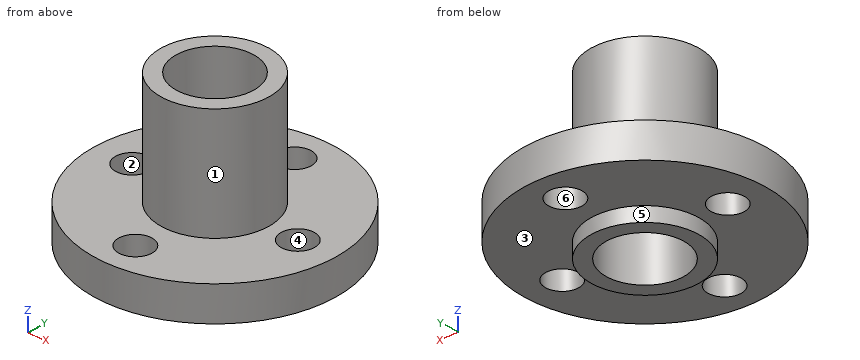
Autodesk Fusion 360 part; units mm, degrees
sketch "Sketch1" plane through (0, 0, 0) normal (0, 0, 1) x (1, 0, 0)
  circle A0 centre (0, 0) radius 10.9
  dimension "d1" = 21.8
extrude "Extrude1" add sketch "Sketch1" along normal blind 3.1
sketch "Sketch2" plane through (0, 0, 3.1) normal (0, 0, 1) x (-1, 0, 0)
  circle A0 centre (0, 0) radius 10.9
  circle A1 centre (0, 0) radius 4.85
  dimension "d4" = 9.7
extrude "Extrude2" add sketch "Sketch2" along normal blind 10 contours A1
sketch "Sketch3" plane through (0, 0, 0) normal (0, 0, 1) x (1, 0, 0)
  circle A0 centre (0, 0) radius 4.85
  dimension "d7" = 9.7
extrude "Extrude3" add sketch "Sketch3" against normal blind 1.3
sketch "Sketch4" plane through (0, 0, 13.1) normal (0, 0, 1) x (-1, 0, 0)
  circle A0 centre (0, 0) radius 4.85
  circle A1 centre (0, 0) radius 3.5
  dimension "d10" = 7
extrude "Extrude4" cut sketch "Sketch4" against normal through all contours A1
thread "Thread1" thread offset 0 thread length 10
sketch "Sketch5" plane through (0, 0, 3.1) normal (0, 0, 1) x (-1, 0, 0)
  circle A0 centre (0, 0) radius 4.85
  circle A1 centre (0, 0) radius 10.9
  line L0 (-10.9, 0) -> (10.9, 0) construction
  circle A2 centre (7.5, 0) radius 1.5
  circle A3 centre (7.5, 0) radius 1.5
  dimension "d14" = 3
  dimension "d18" = 3
extrude "Extrude5" cut sketch "Sketch5" against normal through all contours A2 A3
mirror "Mirror1" about plane through (0, 0, 0) normal (1, 0, 0) of "Extrude5"
sketch "Sketch6" plane through (0, 0, 3.1) normal (0, 0, 1) x (-1, 0, 0)
  circle A0 centre (-7.5, 0) radius 1.5
  circle A1 centre (7.5, 0) radius 1.5
  circle A2 centre (0, 0) radius 4.85
  circle A3 centre (0, 0) radius 10.9
  circle A4 centre (0, -7.875) radius 1.5
  line L0 (0, -4.85) -> (0, -10.9) construction
  dimension "d19" = 3
extrude "Extrude6" cut sketch "Sketch6" against normal through all contours A4
mirror "Mirror2" about plane through (0, 0, 0) normal (0, 1, 0) of "Extrude6"
Geometry: final body of the model. Coordinates: model frame, mm. Face numbers are marked on the shaded views. A direction names the side the tool comes from. Coordinates: 2 decimals unless noted, no trailing zeros. Order: outer loops, then holes, each group sorted by start corner. A loop starts at its lowest first (then second) coordinate and runs counter-clockwise, first axis right, second up.
(1) Section query B-B (y = 0.5). Return the cut outline in (x, z), plus the area to 3 significant figures.
(2) First-contact query: pin 1 (6 mm diameter, centred on x = 0, z = 6.5, fed in from -Y); pin 2 (5 mm diameter, centred on y = -2, z = 7.5, fed in from +X); pin 3 (2.5 mm diameter, centred on x = -7.5, y = 0, fed in from +Z); pin 4 (5 mm diameter, centred on x = 0, y = 7.875, fed in from -Z). Flat tips, straight axial feed; report the tip coordinate or a pass-through.
(3) Access query for the marked faces 1 and 2. Directions: +Z, -Z, +X, -X, +Y, -Y. A direction counts if a zero-diameter tool reaches every point of the face in a straight line with its end or side. Return the directions, or none.
(4) Material intervals for probe 1 along Y at (x, z) = (0, 3) (3 decimals); probe 2 along Y at (x, z) = (0, 8.75); probe 3 along Z at (x, y) = (5.75, 8.25), sorted ascending.
(5) Section query A-A (x = 0). Return the cut outline in (y, z) (3 decimals), plus the area to 3 significant figures.
(6) Draft query along Y for the marked faces 3, 4, 5 and 6. Return one class per face: pulls with the +Y half, pulls with the -Y half, needs draft (parallel to the pull), parting line crosses it, or undercut.
(7) Section query D-D (z = 1.25). Return the cut outline in (x, y) (3 decimals), plus the area to 3 significant figures.
(8) Section query C-C (x = 7.5). Return the cut outline in (y, z), plus the area to 3 significant figures.
Solution:
1. outline: (-10.89, 0) - (-8.91, 0) - (-8.91, 3.1) - (-10.89, 3.1) - close; (-6.09, 0) - (-4.82, 0) - (-4.82, -1.3) - (-3.46, -1.3) - (-3.46, 13.1) - (-4.82, 13.1) - (-4.82, 3.1) - (-6.09, 3.1) - close; (3.46, -1.3) - (4.82, -1.3) - (4.82, 0) - (6.09, 0) - (6.09, 3.1) - (4.82, 3.1) - (4.82, 13.1) - (3.46, 13.1) - close; (8.91, 0) - (10.89, 0) - (10.89, 3.1) - (8.91, 3.1) - close
1. area: 59.2 mm2
2. pin 1: stops at y = -4.85
2. pin 2: stops at x = 4.85
2. pin 3: passes through
2. pin 4: stops at z = 0
3. face 1: +Z
3. face 2: +Z, -Z
4. probe 1: y = -10.9 to -9.375, -6.375 to -3.5, 3.5 to 6.375, 9.375 to 10.9
4. probe 2: y = -4.85 to -3.5, 3.5 to 4.85
4. probe 3: z = 0 to 3.1
5. outline: (-10.9, 0) - (-9.375, 0) - (-9.375, 3.1) - (-10.9, 3.1) - close; (-6.375, 0) - (-4.85, 0) - (-4.85, -1.3) - (-3.5, -1.3) - (-3.5, 13.1) - (-4.85, 13.1) - (-4.85, 3.1) - (-6.375, 3.1) - close; (3.5, -1.3) - (4.85, -1.3) - (4.85, 0) - (6.375, 0) - (6.375, 3.1) - (4.85, 3.1) - (4.85, 13.1) - (3.5, 13.1) - close; (9.375, 0) - (10.9, 0) - (10.9, 3.1) - (9.375, 3.1) - close
5. area: 57.8 mm2
6. face 3: needs draft
6. face 4: undercut
6. face 5: parting line crosses it
6. face 6: undercut
7. outline: circle Ø21.8 at (0, 0); hole circle Ø3 at (-7.5, 0); hole circle Ø7 at (0, 0); hole circle Ø3 at (0, -7.875); hole circle Ø3 at (0, 7.875); hole circle Ø3 at (7.5, 0)
7. area: 306 mm2
8. outline: (-7.91, 0) - (-1.5, 0) - (-1.5, 3.1) - (-7.91, 3.1) - close; (1.5, 0) - (7.91, 0) - (7.91, 3.1) - (1.5, 3.1) - close
8. area: 39.7 mm2
